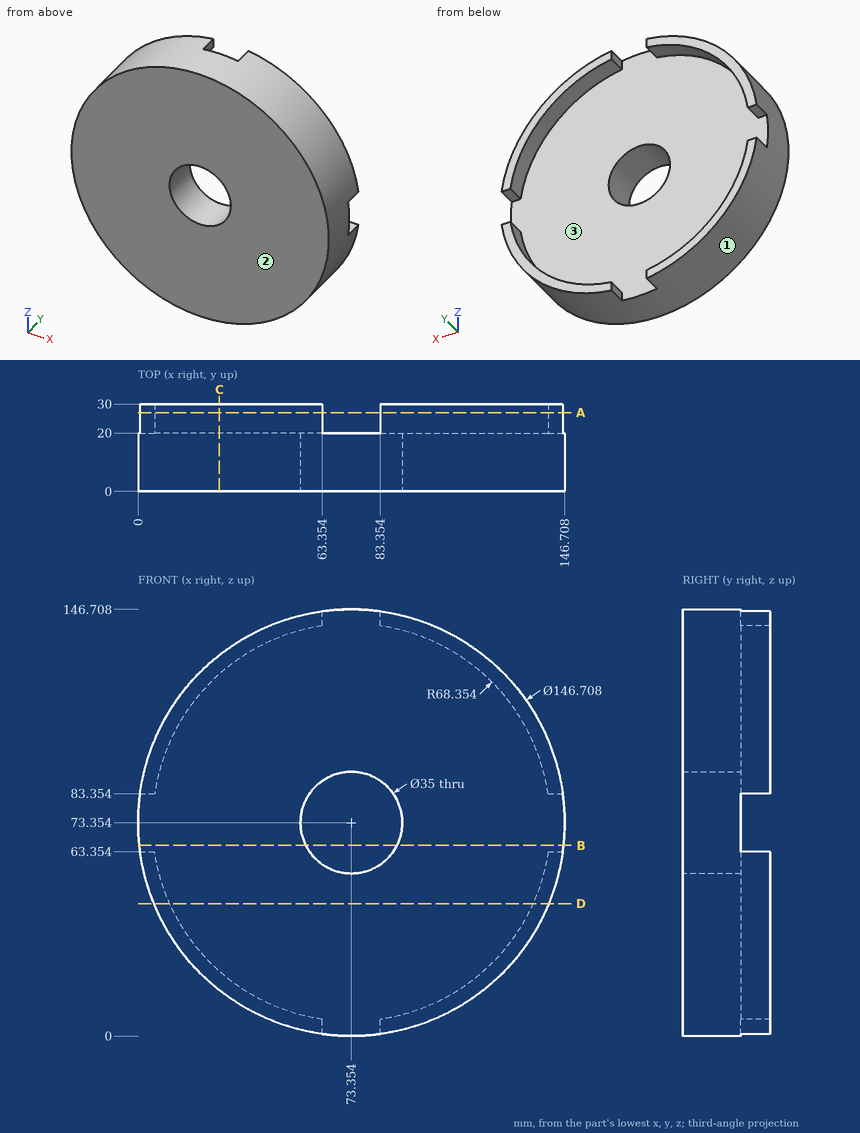
Geometry check sheet. Reference: drawing and pictorial views, mm from the part's lowest x, y, z. Coordinates: 2 decimals unless noted, no trailing zeros. Write each loop counter-clockwise with the first axis right and the second up, starting at its lowest first coordinate (ties: lowest second). Pieces come first, ordered by that corner, then holes.
Item 1: Depth check by flat-ended pin: pin 1 Ø1.5 at (y, z) = (24, 37.5) entering from -X (3 decimals); pin 2 Ø2 at (x, z) = (122, 38.5) entering from +Y; pin 3 Ø5.5 at (x, y) = (3.5, 24.5) entering from +Z. Enter the tip coordinate at first touch or a pass-through.
Numbers:
pin 1: stops at x = 8.945
pin 2: stops at y = 20
pin 3: stops at z = 102.98
Item 2: Cross-section at B-B on z = 65.5. Record the boundary of the cut face in (x, y), then the cut area to 3 significant figures.
Numbers:
outline: (0.42, 0) - (57.72, 0) - (57.72, 20) - (0.42, 20) - close; (88.99, 0) - (146.29, 0) - (146.29, 20) - (88.99, 20) - close
area: 2,290 mm2
Item 3: Cross-section at C-C on x = 28. Record the boundary of the cut face in (y, z).
Numbers:
outline: (0, 15.7) - (30, 15.7) - (30, 22.21) - (20, 22.21) - (20, 124.49) - (30, 124.49) - (30, 131.01) - (0, 131.01) - close
Item 4: Mould release check, pull along Z, two halves, no side actions. Record for the marked faces 1, 2 and 3: released by +Z, released by -Z, zero draft, split by the parting line, or undercut.
Numbers:
face 1: split by the parting line
face 2: zero draft
face 3: undercut
Item 5: Scan lines: probe 1 along Y at (x, z) = (130.5, 81.5); probe 2 along X at (y, z) = (28.25, 96.5); probe 3 along X at (y, z) = (22.25, 41). Record each from-to range of solid material in increasing order.
Numbers:
probe 1: y = 0 to 20
probe 2: x = 3.75 to 9.04, 137.67 to 142.96
probe 3: x = 7.52 to 13.14, 133.57 to 139.19
Item 6: Cross-section at D-D on z = 45.5. Record the boundary of the cut face in (x, y).
Numbers:
outline: (5.49, 0) - (141.21, 0) - (141.21, 30) - (135.78, 30) - (135.78, 20) - (10.93, 20) - (10.93, 30) - (5.49, 30) - close
Item 7: Cross-section at A-A on y = 27. Record the boundary of the cut face in (x, z).
Numbers:
outline: (0.68, 63.35) arc R73.35 ccw to (63.35, 0.68) - (63.35, 5.74) arc R68.35 cw to (5.74, 63.35) - close; (0.68, 83.35) - (5.74, 83.35) arc R68.35 cw to (63.35, 140.97) - (63.35, 146.02) arc R73.35 ccw to start; (83.35, 0.68) arc R73.35 ccw to (146.02, 63.35) - (140.97, 63.35) arc R68.35 cw to (83.35, 5.74) - close; (83.35, 140.97) arc R68.35 cw to (140.97, 83.35) - (146.02, 83.35) arc R73.35 ccw to (83.35, 146.02) - close
